Input: dimensioned drawing with shaded views. Units: mm. Origin: part minimum x, y, z. Give positions to 0.01 mm unless a question says otherwise; leave off trailing zeros. Loops run counter-clockwise (first coordinate to the right, second up) from the corner with the lowest first, then second, coordinate; pieces in that order, holes last.
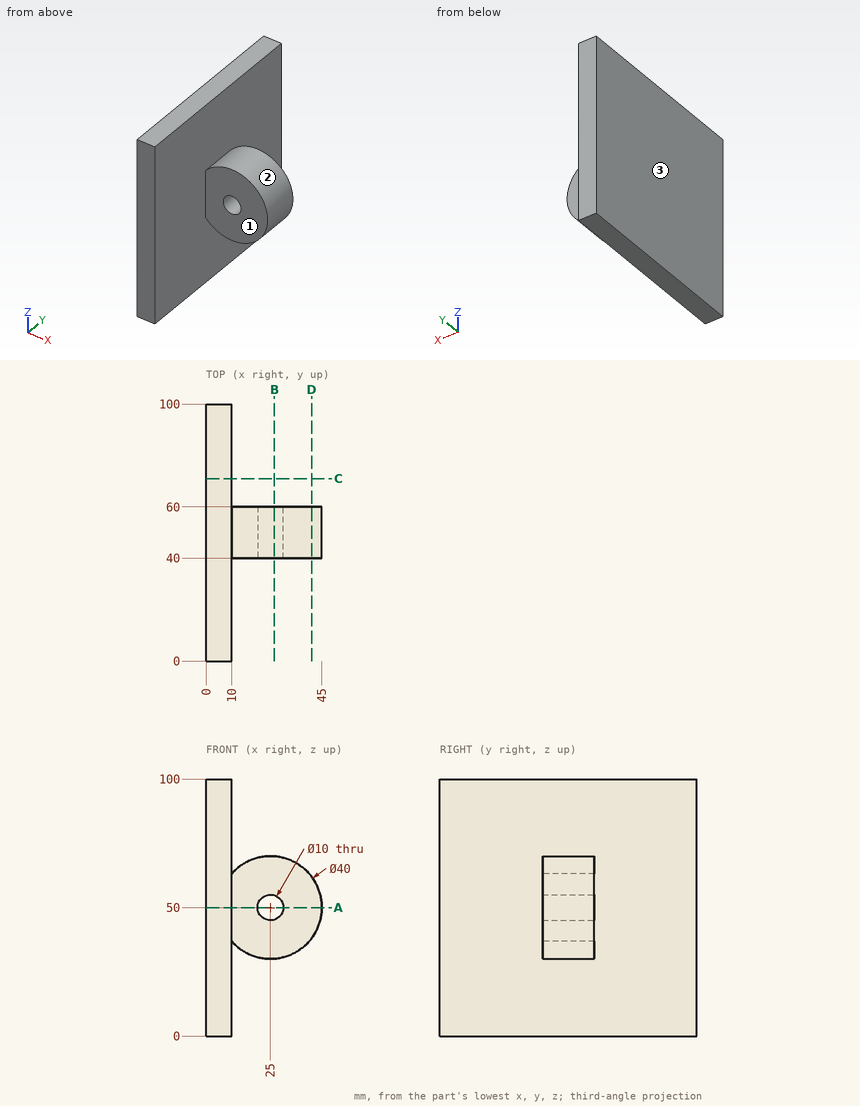
Item 1: Ray query, probe 1 along Z at (x, y) = (25, 46); probe 2 along X at (y, z) = (84, 28); probe 3 along Y at (x, z) = (33.5, 56). Return the intervals inside material, ascending.
Values follow:
probe 1: z = 30 to 45, 55 to 70
probe 2: x = 0 to 10
probe 3: y = 40 to 60
Item 2: Section query A-A on z = 50. Return loops of the section in (x, y), plus the area to 3 significant figures.
Values follow:
outline: (0, 0) - (10, 0) - (10, 40) - (20, 40) - (20, 60) - (10, 60) - (10, 100) - (0, 100) - close; (30, 40) - (45, 40) - (45, 60) - (30, 60) - close
area: 1,500 mm2
Item 3: Section query B-B on x = 26.5. Return loops of the section in (y, z).
Values follow:
outline: (40, 30.06) - (60, 30.06) - (60, 45.23) - (40, 45.23) - close; (40, 54.77) - (60, 54.77) - (60, 69.94) - (40, 69.94) - close
Item 4: Pin query (flat end, axial travel): pin 1 (2 mm diameter, centred on x = 40, z = 48.5, fed in from +Y); pin 2 (12 mm diameter, centred on y = 56.5, z = 10.5, fed in from +X); pin 3 (8 mm diameter, centred on y = 50, z = 60, fed in from +X). Return the tip coordinate at first contact, or that it passes through.
Values follow:
pin 1: stops at y = 60
pin 2: stops at x = 10
pin 3: stops at x = 44.08
Item 5: Section query C-C on y = 71. Return loops of the section in (x, z), plus the area to 3 significant figures.
Values follow:
outline: (0, 0) - (10, 0) - (10, 100) - (0, 100) - close
area: 1,000 mm2
Item 6: Section query D-D on x = 41. Return loops of the section in (y, z).
Values follow:
outline: (40, 38) - (60, 38) - (60, 62) - (40, 62) - close
Item 7: Draft query along X for the marked faces 1, 2 and 3. Return one class per face: +X half, -X half, draft (parallel to the pull), parting line (faces both ways), or undercut.
Values follow:
face 1: draft
face 2: undercut
face 3: -X half
